Source: three-view drawing plus pictorial views. Frame: mm from the lowest corner of the part. Give positions to 0.01 mm unless a question says otherwise; leave off trailing zeros. Order: outer loops, then holes, each group sorted by start corner. A loop starts at its lowest first (then second) coordinate and runs counter-clockwise, first axis right, second up. Notation, with made-up numbers: M 88.25,-21 L 102.25,-21 A27 ccw 102.25,14 Z; hole C -37.5,84 d3. An arc over 180 degrees is marked long. One line per item, written item: value. Start each with the question number.
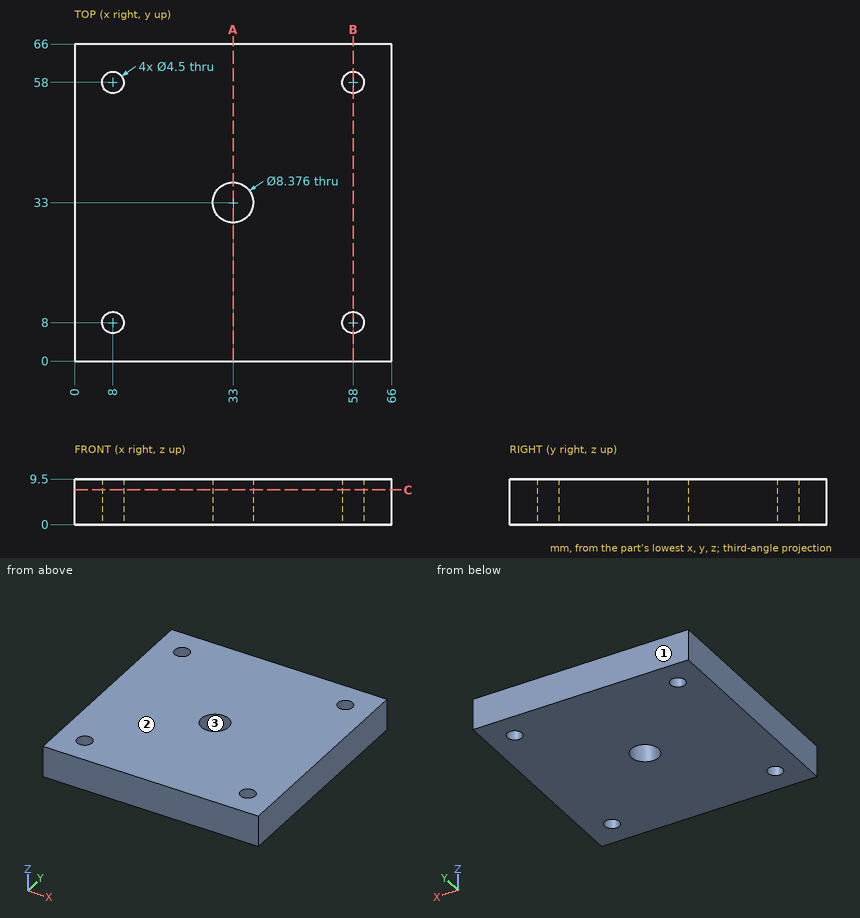
Q1. Ray query, line 1 along X through (y, z) = (8, 5); line 2 along Y through (x, z) = (57, 2). Return the intervals inside material, ascending. Write a range as [from, to].
Q2. Section query C-C on z = 7.25. Return loops of the section in (x, y), and give its area (3 significant figures).
Q3. Section query B-B on x = 58. Return loops of the section in (y, z), and give its area (4 significant figures).
Q4. Mould query, pull axis Y, two halves, no side actions, for the marked faces 1, 2 and 3. Classes: +Y half, -Y half, draft (parallel to the pull), parting line (faces both ways), or undercut.
Q5. Section query A-A on x = 33. Return loops of the section in (y, z).
Results below:
1. line 1: [0, 5.75], [10.25, 55.75], [60.25, 66]
1. line 2: [0, 5.98], [10.02, 55.98], [60.02, 66]
2. outline: M 0,0 L 66,0 L 66,66 L 0,66 Z; hole C 8,8 d4.5; hole C 8,58 d4.5; hole C 33,33 d8.38; hole C 58,8 d4.5; hole C 58,58 d4.5
2. area: 4,240 mm2
3. outline: M 0,0 L 5.75,0 L 5.75,9.5 L 0,9.5 Z; M 10.25,0 L 55.75,0 L 55.75,9.5 L 10.25,9.5 Z; M 60.25,0 L 66,0 L 66,9.5 L 60.25,9.5 Z
3. area: 541.5 mm2
4. face 1: +Y half
4. face 2: draft
4. face 3: undercut
5. outline: M 0,0 L 28.81,0 L 28.81,9.5 L 0,9.5 Z; M 37.19,0 L 66,0 L 66,9.5 L 37.19,9.5 Z
